```python
from build123d import *

# Parameters (mm, degrees)
SKETCH_1_W          = 200
SKETCH_1_H          = 180
EXTRUDE_3_DEPTH     = 35
SKETCH_1_3_W        = 50
SKETCH_1_3_H        = 40
CUT_EXTRUDE_2_DEPTH = 140.014387745
SKETCH_4_W          = 110
SKETCH_4_H          = 100
EXTRUDE_4_DEPTH     = 27.474741722
EXTRUDE_START       = -67.474742
SKETCH_4_4_W        = 110
SKETCH_4_4_H        = 100
EXTRUDE_5_DEPTH     = 25
SKETCH_9_W          = 30
SKETCH_9_H          = 29
CUT_EXTRUDE_5_DEPTH = 247.221445045
CUT_EXTRUDE_6_DEPTH = 27.474741722
SKETCH_11_W         = 34
SKETCH_11_H         = 34
CUT_EXTRUDE_7_DEPTH = 25


with BuildPart() as part:
    # Эскиз1 → Бобышка-Вытянуть3 (new body)
    with BuildSketch(Plane.XY):
        Rectangle(SKETCH_1_W, SKETCH_1_H)
    extrude(amount=EXTRUDE_3_DEPTH)

    # Эскиз1<3> → Вырез-Вытянуть2 (cut, through all)
    with BuildSketch(Plane.XY):
        with BuildLine():
            ThreePointArc((40, -90), (65, -65), (90, -90))
            Line((90, -90), (40, -90))
        make_face()
        with Locations((75, 42.525258278)):
            Rectangle(SKETCH_1_3_W, SKETCH_1_3_H)
    extrude(amount=CUT_EXTRUDE_2_DEPTH, mode=Mode.SUBTRACT)

    # Эскиз4 → Бобышка-Вытянуть4 (add)
    with BuildSketch(Plane(origin=(0, 90, 0), x_dir=(1, 0, 0), z_dir=(0, 1, 0))):
        with Locations((-5, -85)):
            Rectangle(SKETCH_4_W, SKETCH_4_H)
    extrude(amount=-EXTRUDE_4_DEPTH)

    # Эскиз4<4> → Бобышка-Вытянуть5 (add)
    with BuildSketch(Plane(origin=(0, 90, 0), x_dir=(1, 0, 0), z_dir=(0, 1, 0)).offset(EXTRUDE_START)):
        with Locations((-5, -85)):
            Rectangle(SKETCH_4_4_W, SKETCH_4_4_H)
    extrude(amount=-EXTRUDE_5_DEPTH)

    # Эскиз9 → Вырез-Вытянуть5 (cut, through all)
    with BuildSketch(Plane(origin=(0, 90, 0), x_dir=(1, 0, 0), z_dir=(0, 1, 0))):
        with Locations((-85, -14.5)):
            Rectangle(SKETCH_9_W, SKETCH_9_H)
    extrude(amount=-CUT_EXTRUDE_5_DEPTH, mode=Mode.SUBTRACT)

    # Эскиз10 → Вырез-Вытянуть6 (cut)
    with BuildSketch(Plane(origin=(0, 90, 0), x_dir=(1, 0, 0), z_dir=(0, 1, 0))):
        with BuildLine():
            Line((50, -48), (50, -102))
            ThreePointArc((50, -102), (23, -75), (50, -48))
        make_face()
    extrude(amount=-CUT_EXTRUDE_6_DEPTH, mode=Mode.SUBTRACT)

    # Эскиз11 → Вырез-Вытянуть7 (cut)
    with BuildSketch(Plane.XZ.offset(2.474741722)):
        with Locations((33, 65)):
            Rectangle(SKETCH_11_W, SKETCH_11_H)
    extrude(amount=-CUT_EXTRUDE_7_DEPTH, mode=Mode.SUBTRACT)


solid = part.part
```
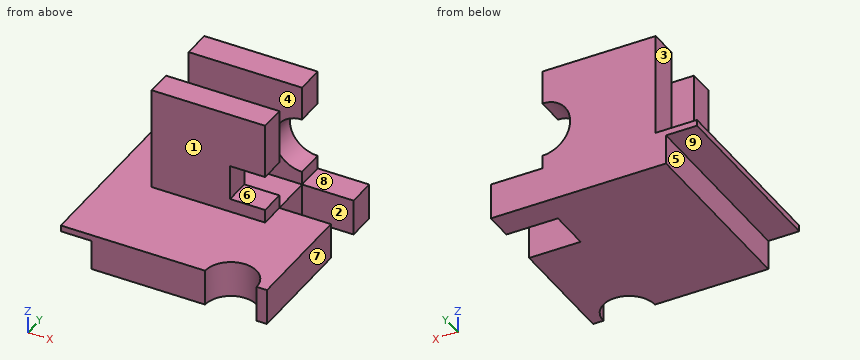
Read the model definition and answer for the solid it produces. Units are mm, in the model's axes. Face numbers are marked on the shaded views. A direction names the side the tool comes from. Give positions to 0.01 mm unless a question says otherwise; leave off trailing zeros. Write each loop counter-clockwise with the first axis right and the second up, starting at its lowest first coordinate (ties: lowest second). Pieces come first, ordered by that corner, then holes. Notation, with made-up numbers: (13.25, -21) - (39.25, -21) arc R5 ccw to (39.25, -17) - close; hole circle Ø5 at (48, 16). An arc over 180 degrees is marked (long way). Write item = value, one per line. Start each with the question number.
Item 1: Each of these flat-tipped pins is pushed along its axis until it touches: P1, Ø3, axis at x = 76, y = 10, coming from the +Z side; P2, Ø9, axis at x = -86.5, y = 38.5, coming from the -Z side; P3, Ø8, axis at y = 74.5, z = 116, coming from the +X side. Where does it stop, or does it pass through?
Item 2: The mould has two halves that part along Z. Classify the marked faces 6, 7, 8 and 9: +Z half, -Z half, draft (parallel to the pull), parting line (faces both ways), or undercut.
Item 3: Find section C-C (y = -29.5). Give the vertices of the cut face in (x, z), then the cut area to 3 significant figures.
Item 4: Find section D-D (x = -33.5). Give the vertices of the cut face in (y, z).
Item 5: Find the intervals of material crossed by probe 1 along Y at (x, z) = (-43.5, 48); probe 2 along Z at (x, y) = (11.5, 47); probe 3 along X at (y, z) = (4.5, 62.5), in increasing order. Write a range as [from, to].
Item 6: Find section B-B (x = 65). Give the vertices of the cut face in (y, z), then the cut area to 4 significant figures.
Item 7: A tool of negligible diameter and unlimited length cuts with its end or side. For the marked faces 1, 2, 3, 4 and 5, from which of +Z, -Z, +X, -X, +Y, -Y can it reach the whole face along a straight path? Write none if from no direction.
Item 8: Find section A-A (z = 75). Give the vertices of the cut face in (x, y).
Response:
q1.P1 = 35
q1.P2 = 29
q1.P3 = 50
q2.face_6 = undercut
q2.face_7 = draft
q2.face_8 = +Z half
q2.face_9 = -Z half
q3.outline = (-100, 29) - (-70, 29) - (-70, 0) - (100, 0) - (100, 35) - (-100, 35) - close
q3.area = 6,130 mm²
q4.outline = (-90, 0) - (90, 0) - (90, 135) - (62.53, 135) - (62.53, 35) - (22.53, 35) - (22.53, 135) - (-2.47, 135) - (-2.47, 35) - (-90, 35) - close
q5.probe_1 = [-2.47, 22.53], [62.53, 90]
q5.probe_2 = [0, 35]
q5.probe_3 = [-60, 16]
q6.outline = (-65, 0) - (22.53, 0) - (22.53, 35) - (-65, 35) - close; (62.53, 0) - (90, 0) - (90, 35) - (62.53, 35) - close
q6.area = 4,025 mm²
q7.face_1 = +Z, +X, -X, -Y
q7.face_2 = +Z, -Z, +X
q7.face_3 = +Z, -X, +Y, -Y
q7.face_4 = +Z, +X, -X
q7.face_5 = -Z, -X, +Y, -Y
q8.outline = (-60, -2.47) - (16, -2.47) - (16, 22.53) - (-60, 22.53) - close; (-60, 62.53) - (23, 62.53) - (23, 90) - (-60, 90) - close
